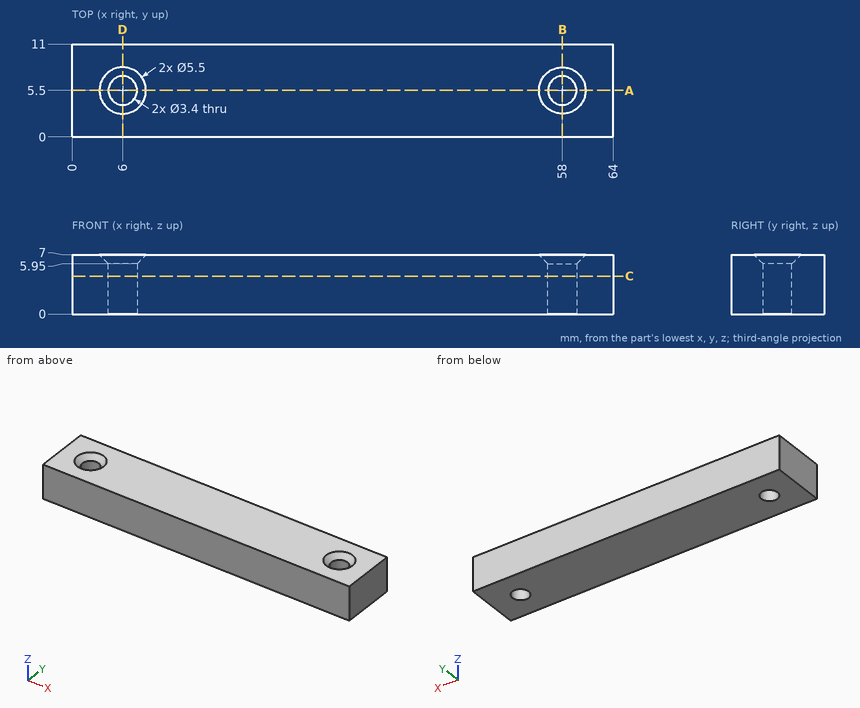
The drawing under review shows one solid part. Ordinate dimensions are in mm from its lowest x, y, z. Round coordinates to 2 decimals unless told otherwise and drop trailing zeros. Loops run counter-clockwise (first coordinate to the right, second up) from the corner with the lowest first, then second, coordinate; pieces in that order, holes last.
Item 1: Take a section at C-C (z = 4.5). Write out the cut boundary in (x, y), then the cut area to 3 significant figures.
Determined:
outline: (0, 0) - (64, 0) - (64, 11) - (0, 11) - close; hole circle Ø3.4 at (6, 5.5); hole circle Ø3.4 at (58, 5.5)
area: 686 mm2
Item 2: Take a section at A-A (y = 5.5). Write out the cut boundary in (x, z), then the cut area to 3 significant figures.
Determined:
outline: (0, 0) - (4.3, 0) - (4.3, 5.95) - (3.25, 7) - (0, 7) - close; (7.7, 0) - (56.3, 0) - (56.3, 5.95) - (55.25, 7) - (8.75, 7) - (7.7, 5.95) - close; (59.7, 0) - (64, 0) - (64, 7) - (60.75, 7) - (59.7, 5.95) - close
area: 398 mm2
Item 3: Take a section at B-B (x = 58). Write out the cut boundary in (y, z).
Determined:
outline: (0, 0) - (3.8, 0) - (3.8, 5.95) - (2.75, 7) - (0, 7) - close; (7.2, 0) - (11, 0) - (11, 7) - (8.25, 7) - (7.2, 5.95) - close
Item 4: For line 1 (Y direction, x = 6, z = 1.8); line 2 (X direction, y = 5, z = 2.75); line 3 (X direction, y = 5.75, z = 1), list the stretches that pass through material, from the lowest coordinate up.
Determined:
line 1: y = 0 to 3.8, 7.2 to 11
line 2: x = 0 to 4.38, 7.62 to 56.38, 59.62 to 64
line 3: x = 0 to 4.32, 7.68 to 56.32, 59.68 to 64
